from build123d import *

# Parameters (mm, degrees)
F1_DEPTH = 38.1
F2_R     = 3.175
F3_DEPTH = 25.4
F4_R     = 2.53999
F5_R     = 2.54
F6_R     = 3.175
F7_DEPTH = 1.5875
F8_R     = 15.875
F8_R_2   = 7.9375
F9_DEPTH = 3.175


# Not quite as in the source:
# - a fillet or chamfer is up to 0.001 mm smaller than in the source, because OpenCascade refuses the exact size
# - a feature names something its author has since deleted; it is built from what else it names


with BuildPart() as f1:
    # F0 (on Front) → F1 (new body)
    with BuildSketch(Plane.XZ):
        with BuildLine():
            ThreePointArc((-15.875, -44.45), (0, -28.575), (15.875, -44.45))
            Line((15.875, -44.45), (15.875, 0))
            ThreePointArc((15.875, 0), (15.0603473566, -5.0201157855), (12.7, -9.525))
            Line((12.7, -9.525), (12.7, -30.2509683429))
            ThreePointArc((12.7, -30.2509683429), (0, -25.4), (-12.7, -30.2509683429))
            Line((-12.7, -30.2509683429), (-12.7, -9.525))
            ThreePointArc((-12.7, -9.525), (-15.0603473566, -5.0201157855), (-15.875, 0))
            Line((-15.875, 0), (-15.875, -44.45))
        make_face()
        with BuildLine():
            ThreePointArc((12.7, -9.525), (15.0603473566, -5.0201157855), (15.875, 0))
            ThreePointArc((15.875, 0), (0, 15.875), (-15.875, 0))
            ThreePointArc((-15.875, 0), (-15.0603473566, -5.0201157855), (-12.7, -9.525))
            ThreePointArc((-12.7, -9.525), (-9.8507599619, -12.4490221774), (-6.35, -14.5496778315))
            Line((-6.35, -14.5496778315), (-6.35, -20.8996778315))
            Line((-6.35, -20.8996778315), (6.35, -20.8996778315))
            Line((6.35, -20.8996778315), (6.35, -14.5496778315))
            ThreePointArc((6.35, -14.5496778315), (9.8507599619, -12.4490221774), (12.7, -9.525))
        make_face()
        with BuildLine():
            Line((-3.175, -18.6467221242), (-3.175, -12.2967221242))
            ThreePointArc((-3.175, -12.2967221242), (0, 12.7), (3.175, -12.2967221242))
            Line((3.175, -12.2967221242), (3.175, -18.6467221242))
            Line((3.175, -18.6467221242), (-3.175, -18.6467221242))
        make_face(mode=Mode.SUBTRACT)
    extrude(amount=F1_DEPTH)

    # F2 (on Right) → F3 (cut, symmetric)
    with BuildSketch(Plane.YZ):
        with Locations((-31.75, -22.86)):
            Circle(F2_R)
        with Locations((-6.35, -22.86)):
            Circle(F2_R)
    extrude(amount=F3_DEPTH, both=True, mode=Mode.SUBTRACT)

    # F4 (radius 2.54 in the source; OpenCascade refuses exactly that, so slightly less here)
    f4_edges = [f1.edges().sort_by_distance(p)[0] for p in [
        (15.875, -19.05, -44.45),
        (-15.875, -19.05, -44.45),
    ]]
    fillet(f4_edges, radius=F4_R)

    # F5
    f5_edges = [f1.edges().sort_by_distance(p)[0] for p in [
        (-15.875, -9.525, -22.86),
        (-15.875, -34.925, -22.86),
        (15.875, -34.925, -22.86),
        (15.875, -9.525, -22.86),
    ]]
    fillet(f5_edges, radius=F5_R)

    # F6 (on face) → F7 (join)
    with BuildSketch(Plane.XZ.offset(38.1)):
        with BuildLine():
            ThreePointArc((6.35, -14.5496778315), (0, 15.875), (-6.35, -14.5496778315))
            Line((-6.35, -14.5496778315), (-6.35, -20.8996778315))
            Line((-6.35, -20.8996778315), (6.35, -20.8996778315))
            Line((6.35, -20.8996778315), (6.35, -14.5496778315))
        make_face()
        Circle(F6_R, mode=Mode.SUBTRACT)
    extrude(amount=-F7_DEPTH)

    # F8 (on face) → F9 (join)
    with BuildSketch(Plane.XZ.offset(38.1)):
        Circle(F8_R)
        Circle(F8_R_2, mode=Mode.SUBTRACT)
    extrude(amount=F9_DEPTH)


solid = f1.part
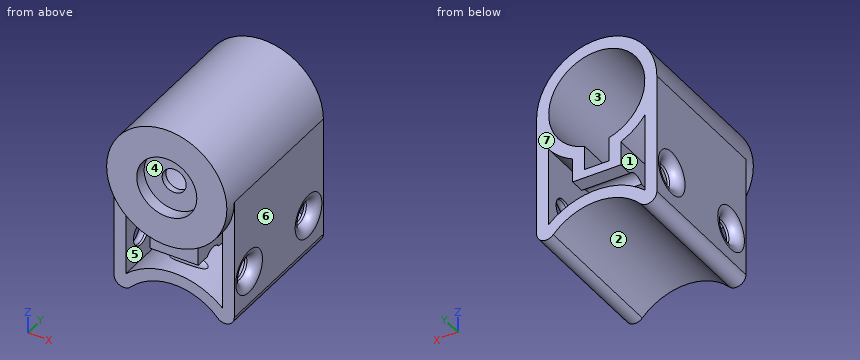
Input: part model. Units: mm. Frame: model coordinates. Face numbers are marked on the shaded views. A direction names the side the tool comes from. Coordinates: 2 decimals unless noted, no trailing zeros. Loops run counter-clockwise (first coordinate to the right, second up) from the corner with the lowest first, then second, coordinate; pieces in that order, holes last.
Q1. Material intervals for line 1 (Z direction, x = 0.5, y = -35); line 2 (X direction, y = -25, z = -0.5) (3 decimals); line 3 (X direction, y = -27, z = -14) (3 decimals), sorted ascending.
Q2. Cut plane C-C (y = -23). Output: boundary loops of the cut face in (x, z) (3 decimals).
Q3. Draft query along X for the marked faces 5, 6 and 7. Return one class per face: +X half, -X half, draft (parallel to the pull), parting line (faces both ways), or undercut.
Q4. Cut plane D-D (x = -9). Output: boundary loops of the cut face in (y, z) (1 decimal), then the cut area to 3 significant figures.
Q5. Set-up query: the marked faces 1, 2, 3 and 4. Return all of +Z, -Z, +X, -X, +Y, -Y with unobstructed straight access to the full face (end or side cutting, diameter ignored); none if empty.
Q6. Contact query for flat-ended pins moving along their axis: pin 1 (9.5 mm diameter, centred on x = 0, z = 0, fed in from -Y); pin 2 (4 mm diameter, centred on y = -6.35, z = -22.86, fed in from +X); pin 3 (10 mm diameter, centred on x = -4.5, y = -12.5, fed in from -Z); pin 4 (14 mm diameter, centred on x = 0.5, y = -21, fed in from -Z). Output: stop coordinate, or through.
Q7. Cut plane A-A (y = -31.75). Give the number of separate pieces and of enclosed holes in the cut face, then the cut area to 3 significant figures.
Working result:
1. line 1: z = -28.58 to -25.41, -20.9 to -18.65, 12.69 to 15.87
1. line 2: x = -15.875 to -12.69, 12.69 to 15.875
1. line 3: x = -15.875 to -12.7, -7.484 to -3.175, 3.175 to 7.484, 12.7 to 15.875
2. outline: (-15.875, -31.75) arc R2.54 ccw to (-11.496, -33.502) arc R15.875 cw to (11.496, -33.502) arc R2.54 ccw to (15.875, -31.75) - (15.875, 0) arc R15.875 ccw to (-15.875, 0) - close; hole (-12.7, -30.251) arc R19.05 cw to (12.7, -30.251) - (12.7, -9.525) arc R15.875 cw to (6.35, -14.55) - (6.35, -20.9) - (-6.35, -20.9) - (-6.35, -14.55) arc R15.875 cw to (-12.7, -9.525) - close; hole (-3.175, -18.647) - (3.175, -18.647) - (3.175, -12.297) arc R12.7 ccw (long way) to (-3.175, -12.297) - close
3. face 5: undercut
3. face 6: +X half
3. face 7: draft
4. outline: (-41.3, -13.1) - (0, -13.1) - (0, -9) - (-36.5, -9) - (-36.5, 9) - (0, 9) - (0, 13.1) - (-41.3, 13.1) - close; (-38.1, -31.4) - (0, -31.4) - (0, -27.7) - (-38.1, -27.7) - close
4. area: 567 mm2
5. face 1: +Y, -Y
5. face 2: -Z, +Y, -Y
5. face 3: +Y
5. face 4: -Y
6. pin 1: stops at y = -38.1
6. pin 2: passes through
6. pin 3: stops at z = -31.73
6. pin 4: stops at z = -30.46
7. separate pieces: 2
7. enclosed holes: 1
7. area: 514 mm2
